Autodesk Inventor part; units mm, degrees
ref_plane "Work Plane1" through (-13, 0, -15) normal (0, 0, 1) x (1, 0, 0)
ref_plane "Work Plane2" through (0, 2.25, 0) normal (0, 1, 0) x (-1, 0, 0)
ref_plane "YZ Plane" through (0, 0, 0) normal (1, 0, 0) x (0, 1, 0)
sketch "Sketch1" plane through (0, 0, 0) normal (0, 1, 0) x (-1, 0, 0)
  line L0 (64, 0) -> (-64, 0)
  line L1 (-64, 0) -> (-64, -30)
  line L2 (-64, -30) -> (64, -30)
  line L3 (64, -30) -> (64, 0)
  line L4 (13, -15) -> (-13, -15) construction
  line L5 (13, -7.5) -> (-13, -7.5)
  line L6 (-13, -22.5) -> (13, -22.5)
  arc A0 (13, -22.5) -> (13, -7.5) centre (13, -15) ccw
  arc A1 (-13, -7.5) -> (-13, -22.5) centre (-13, -15) ccw
  line L7 (13, -15) -> (64, -15) construction
  line L8 (0, -15) -> (0, -30) construction
  point P0 (0, 0)
  point P1 (0, 0)
  dimension "d0" = 128
  dimension "d1" = 30
  dimension "d2" = 15
  dimension "d3" = 26
extrude "Extrusion1" add sketch "Sketch1" along normal blind 4.5
sketch "Sketch2" plane through (0, 4.5, 0) normal (0, 1, 0) x (1, 0, 0)
  arc A0 (-13, 22.5) -> (-13, 7.5) centre (-13, 15) ccw construction
  line L0 (-13, 22.5) -> (13, 22.5) construction
  arc A1 (13, 7.5) -> (13, 22.5) centre (13, 15) ccw construction
  line L1 (13, 7.5) -> (-13, 7.5) construction
  line L2 (-64, 0) -> (64, 0) construction
  line L3 (64, 0) -> (64, 30) construction
  line L4 (64, 30) -> (-64, 30) construction
  line L5 (-64, 30) -> (-64, 0) construction
  line L6 (-64, 20.25) -> (-59.5, 20.25)
  line L7 (-59.5, 20.25) -> (-59.5, 16.75)
  line L8 (-59.5, 16.75) -> (-55.5, 16.75)
  line L9 (-55.5, 16.75) -> (-55.5, 18)
  line L10 (-55.5, 18) -> (-52.5, 18)
  line L11 (-52.5, 18) -> (-52.5, 16.75)
  line L12 (-52.5, 16.75) -> (-47.5, 16.75)
  line L13 (-47.5, 16.75) -> (-47.5, 13.25)
  line L14 (-47.5, 13.25) -> (-52.5, 13.25)
  line L15 (-52.5, 13.25) -> (-52.5, 12)
  line L16 (-52.5, 12) -> (-55.5, 12)
  line L17 (-55.5, 12) -> (-55.5, 13.25)
  line L18 (-55.5, 13.25) -> (-59.5, 13.25)
  line L19 (-59.5, 9.75) -> (-64, 9.75)
  line L20 (-59.5, 9.75) -> (-59.5, 13.25)
  line L21 (-64, 15) -> (-47.5, 15) construction
  line L22 (-64, 20.25) -> (-64, 9.75)
  line L23 (-64, 30) -> (-64, 0)
  dimension "d6" = 10.5
  dimension "d7" = 4
  dimension "d8" = 3
  dimension "d9" = 5
  dimension "d10" = 3.5
  dimension "d11" = 6
  dimension "d12" = 4.5
extrude "Extrusion2" cut sketch "Sketch2" against normal through all
mirror "Mirror1" about plane through (0, 0, 0) normal (1, 0, 0) of "Extrusion2"
ref_plane "Work Plane1" through (-13, 0, -15) normal (0, 0, 1) x (1, 0, 0)
ref_plane "Work Plane2" through (0, 2.25, 0) normal (0, 1, 0) x (-1, 0, 0)
equation "\"d16\" = 0.5 * THICKNESS"
properties part number "A8-0006"
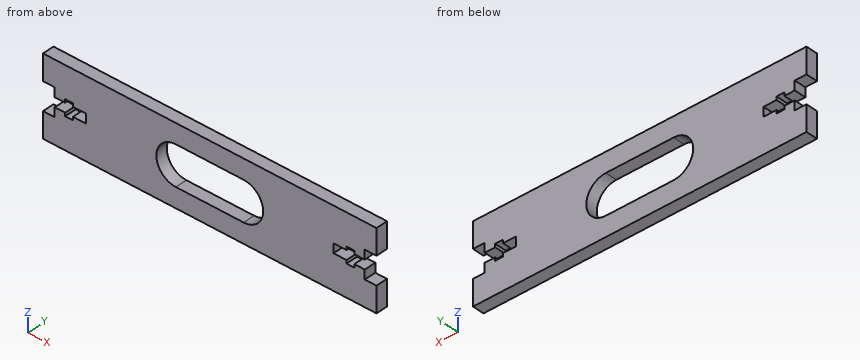
The model under review builds one solid part; all positions refer to its coordinate system, in mm. Give positions to 0.01 mm unless a question says otherwise; leave off trailing zeros. Loops run counter-clockwise (first coordinate to the right, second up) from the corner with the lowest first, then second, coordinate; pieces in that order, holes last. Notation, with made-up numbers: (1, -9) - (22, -9) arc R5 cw to (22, -4) - close; hole circle Ø11 at (0, 54.25). An arc over 180 degrees is marked (long way). Answer as a JSON object with one key per item and string values.
Q1. Add section A-A on z = -15. State the section outline as (x, y) points, plus the area to 3 significant figures.
Worked out:
{"outline": "(-47.5, 0) - (-20.5, 0) - (-20.5, 4.5) - (-47.5, 4.5) - close; (20.5, 0) - (47.5, 0) - (47.5, 4.5) - (20.5, 4.5) - close", "area": "243 mm^2"}
Q2. To check wall thickness, follow line 1 along Z through (x, y) = (12, 3.1); line 2 along X through (y, z) = (3.4, -17.75); line 3 along Z through (x, y) = (53, 3.2). State the ranges of each line that lie inside material, in increasing order.
Worked out:
{"line 1": "z = -30 to -22.5, -7.5 to 0", "line 2": "x = -59.5 to -55.5, -52.5 to -19.98, 19.98 to 52.5, 55.5 to 59.5", "line 3": "z = -30 to -18, -12 to 0"}
Q3. Insertion check: pin 1 (1.8 mm diameter, centred on y = 2.5, z = -19, fed in from +X); pin 2 (1 mm diameter, centred on y = 2.5, z = -19, fed in from -X). Each pin has a flat end and moves straight along its axis. Give the tip position at first contact, or say it passes through.
Worked out:
{"pin 1": "stops at x = 59.5", "pin 2": "stops at x = -59.5"}
Q4. Add section B-B on x = -10.5. State the section outline as (y, z) points, plus the area to 3 significant figures.
Worked out:
{"outline": "(0, -30) - (4.5, -30) - (4.5, -22.5) - (0, -22.5) - close; (0, -7.5) - (4.5, -7.5) - (4.5, 0) - (0, 0) - close", "area": "67.5 mm^2"}
